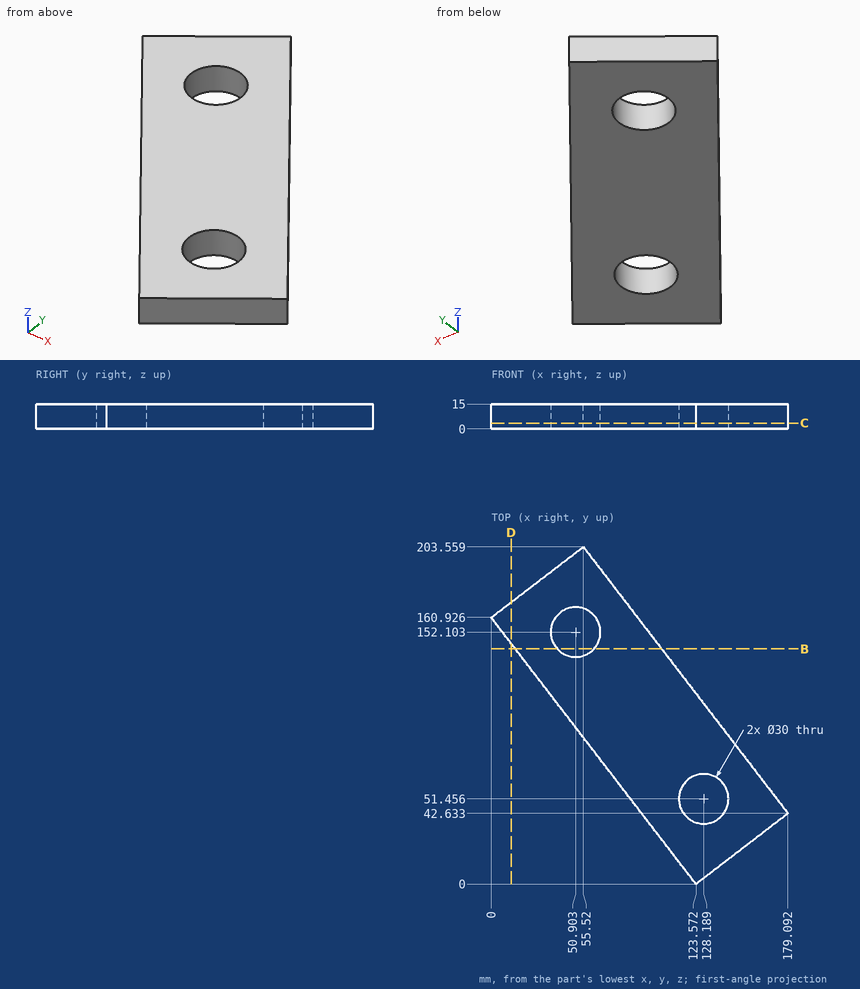
Here's the drawing with two shaded views (mm, measured from the low corner). I have some questions. Give positions to 0.01 mm unless a question says otherwise; leave off trailing zeros. Loops run counter-clockwise (first coordinate to the right, second up) from the corner with the lowest first, then second, coordinate; pieces in that order, holes last. Notation, with made-up numbers: (-17.5, 84.25) -> (-12.5, 84.25) arc R24 cw to (-12.5, 108.25) -> close; hole circle Ø3 at (80.5, 19.25). An arc over 180 degrees is marked (long way). Use one line per item in the form item = value.
1) If we section it at D-D (x = 12): Please give me the cut outline in (y, z), plus the area to 3 significant figures.
Answers:
outline = (145.3, 0) -> (170.14, 0) -> (170.14, 15) -> (145.3, 15) -> close
area = 373 mm²
2) Will these pins go through, and if not, where does the flat tip stop? pin 1 (3 mm diameter, centred on y = 100, z = 3.5, fed in from -X); pin 2 (5 mm diameter, centred on x = 54, z = 8.5, fed in from -Y); pin 3 (4 mm diameter, centred on x = 34, z = 13, fed in from +Y).
Answers:
pin_1 = 45.63
pin_2 = 87.35
pin_3 = 188.57
3) If we section it at B-B (y = 142): Please give me the cut outline in (x, z), plus the area to 3 significant figures.
Answers:
outline = (14.53, 0) -> (39.82, 0) -> (39.82, 15) -> (14.53, 15) -> close; (61.99, 0) -> (102.79, 0) -> (102.79, 15) -> (61.99, 15) -> close
area = 991 mm²
4) If we section it at C-C (z = 3.5): Please give me the cut outline in (x, y) (1 decimal).
Answers:
outline = (0, 160.9) -> (123.6, 0) -> (179.1, 42.6) -> (55.5, 203.6) -> close; hole circle Ø30 at (50.9, 152.1); hole circle Ø30 at (128.2, 51.5)
5) I need wall thicknesses on line 1 along Y through (x, z) = (62, 4.25) (1 decimal); line 2 along Y through (x, z) = (64.5, 1.75) (1 decimal); line 3 along X through (y, z) = (44, 11) (1 decimal). Which ranges of each line are inside material? Lowest first, please.
Answers:
line_1 = 80.2 to 142, 162.2 to 195.1
line_2 = 76.9 to 145.8, 158.4 to 191.9
line_3 = 89.8 to 115.2, 141.2 to 178
